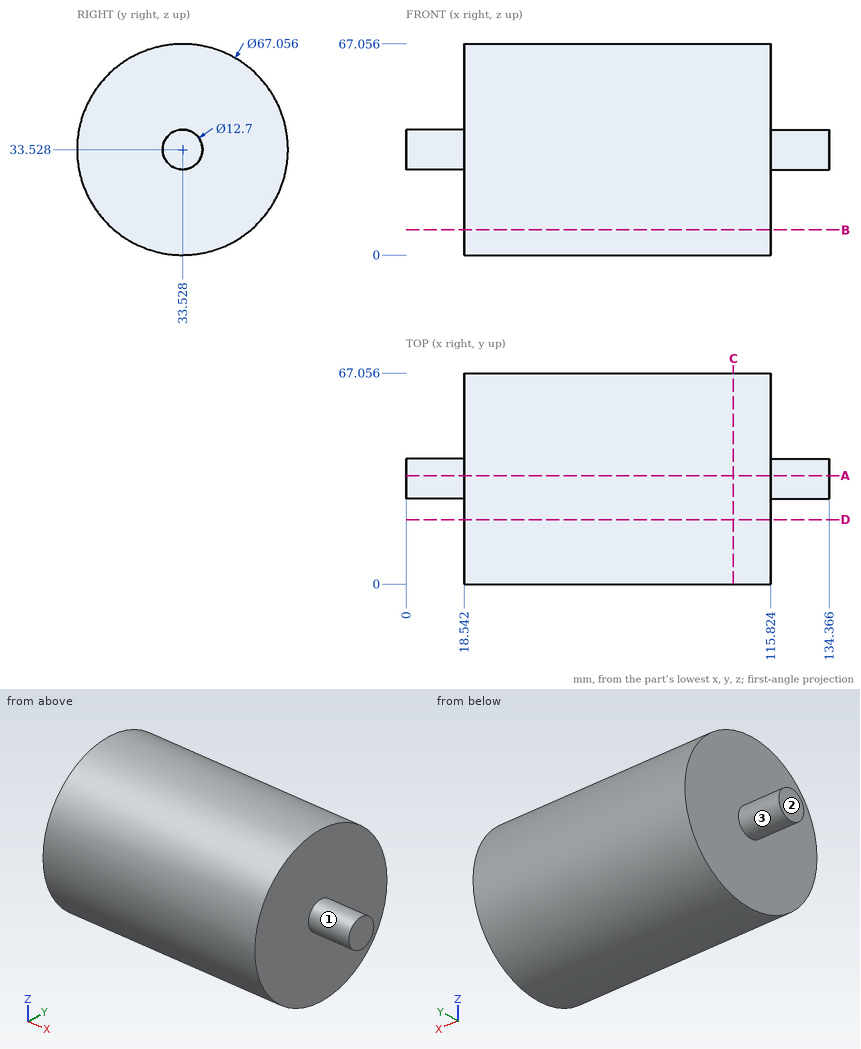
Design review of the part shown in the three views and the two pictorial views. Dimensions are in mm from the part's minimum x, y and z. A direction names the side the tool comes from. Coordinates: 2 decimals unless noted, no trailing zeros. Loops run counter-clockwise (first coordinate to the right, second up) from the corner with the lowest first, then second, coordinate; pieces in that order, holes last.
Q1. We need section A-A on y = 34.5. State the section outline as (x, z) points, and give its area (3 significant figures).
Reported:
outline: (0, 27.25) - (18.54, 27.25) - (18.54, 0.01) - (115.82, 0.01) - (115.82, 27.25) - (134.37, 27.25) - (134.37, 39.8) - (115.82, 39.8) - (115.82, 67.04) - (18.54, 67.04) - (18.54, 39.8) - (0, 39.8) - close
area: 6,990 mm2
Q2. Tool access review of the marked faces 1, 2 and 3: name each direction out of +Z, -Z, +X, -X, +Y, -Y from which nothing blocks a thin tool from reaching the whole face with its end or side.
Reported:
face 1: +X
face 2: +Z, -Z, -X, +Y, -Y
face 3: -X
Q3. We need section C-C on x = 104. State the section outline as (y, z) points.
Reported:
outline: circle Ø67.06 at (33.53, 33.53)
Q4. We need section D-D on y = 20.5. State the section outline as (x, z) points, and give its area (3 significant figures).
Reported:
outline: (18.54, 2.63) - (115.82, 2.63) - (115.82, 64.42) - (18.54, 64.42) - close
area: 6,010 mm2
Q5. We need section B-B on z = 8. State the section outline as (x, y) points, and give its area (3 significant figures).
Reported:
outline: (18.54, 11.79) - (115.82, 11.79) - (115.82, 55.26) - (18.54, 55.26) - close
area: 4,230 mm2
Q6. For pin 1 (1 mm diameter, centred on y = 57.5, z = 21, fed in from +X); pin 2 (2 mm diameter, centred on x = 17, z = 59, fed in from +Y); pin 3 (5 mm diameter, centred on y = 39.5, z = 8.5, fed in from -X); pin 4 (4 mm diameter, centred on x = 97.5, z = 9, fed in from +Y), all flat-tipped, find the tip position at first contact; note any pin that passes through.
Reported:
pin 1: stops at x = 115.82
pin 2: passes through
pin 3: stops at x = 18.54
pin 4: stops at y = 58.36
Q7. To check wall thickness, follow line 1 (X direction, y = 23, z = 57); line 2 (Y direction, x = 111, z = 5); line 3 (Y direction, x = 103, z = 45.5). State the ranges of each line that lie inside material, in increasing order.
Reported:
line 1: x = 18.54 to 115.82
line 2: y = 15.91 to 51.14
line 3: y = 2.21 to 64.85
